Geometry: final body of the model. Coordinates: model frame, mm. Coordinates: 2 decimals unless noted, no trailing zeros. Loops run counter-clockwise (first coordinate to the right, second up) from the corner with the lowest first, then second, coordinate; pieces in that order, holes last. Notation, with made-up numbers: (53.5, 75.25) -> (90.5, 75.25) arc R26 cw to (90.5, 113.25) -> close; hole circle Ø7 at (31.25, -6). An arc over 180 degrees is marked (long way). One line per item, written item: value. Start each with the question number.
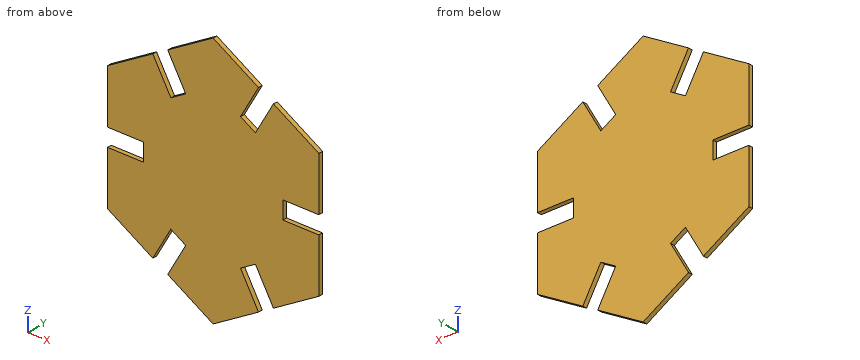
from build123d import *

# Parameters (mm, degrees)
BOSS_EXTRUDE1_DEPTH = 1.5875
SKETCH2_W           = 13.27114317
SKETCH2_H           = 6.35
CUT_EXTRUDE1_DEPTH  = 71.000903906


with BuildPart() as part:
    # Sketch1 → Boss-Extrude1 (new body)
    with BuildSketch(Plane(origin=(0, 0, 0), x_dir=(1, 0, 0), z_dir=(0, 1, 0))):
        Polygon((26.221215583, 24.643793134), (-12.749927587, 47.143793134), (-51.721070757, 24.643793134), (-51.721070757, -20.356206866), (-12.749927587, -42.856206866), (26.221215583, -20.356206866), align=None)
    extrude(amount=BOSS_EXTRUDE1_DEPTH)

    # Sketch2 → Cut-Extrude1 (cut, through all)
    with BuildSketch(Plane(origin=(0, 1.5875, 0), x_dir=(1, 0, 0), z_dir=(0, 1, 0))):
        with Locations((19.585643998, 2.143793134)):
            Rectangle(SKETCH2_W, SKETCH2_H)
        Polygon((2.84970307, 22.813146011), (9.485274655, 34.306293134), (3.986013341, 37.481293134), (-2.649558244, 25.988146011), align=None)
        Polygon((-22.85029693, 25.988146011), (-29.485868515, 37.481293134), (-34.985129829, 34.306293134), (-28.349558244, 22.813146011), align=None)
        with Locations((-45.085499172, 2.143793134)):
            Rectangle(SKETCH2_W, SKETCH2_H)
        Polygon((3.986013341, -33.193706866), (9.485274655, -30.018706866), (2.84970307, -18.525559743), (-2.649558244, -21.700559743), align=None)
        Polygon((-34.985129829, -30.018706866), (-29.485868515, -33.193706866), (-22.85029693, -21.700559743), (-28.349558244, -18.525559743), align=None)
    extrude(amount=-CUT_EXTRUDE1_DEPTH, mode=Mode.SUBTRACT)


solid = part.part
1. Line query: L1, parallel to X at y = 0.4, z = 29; L2, parallel to X at y = 1.15, z = 22; L3, parallel to Z at x = -2, y = 0.9. Output: solid intervals per line, ascending. Write a range as [from, to].
2. Pin query (flat end, axial travel): pin 1 Ø0.5 at (y, z) = (1, -2) entering from +X; pin 2 Ø0.8 at (x, y) = (20.5, 1) entering from +Z; pin 3 Ø0.5 at (x, y) = (19.5, 0.5) entering from -Z. Return the tip coordinate at first contact, or that it passes through.
3. Section D-D on x = -15.5. Return the cut outline in (y, z), plus the area to 3 significant figures.
4. Section C-C on z = -2.5. Return the cut outline in (x, y), plus the area to 3 significant figures.
5. Section B-B on x = 15. Return the cut outline in (y, z), plus the area to 3 significant figures.
Checks:
1. L1: [-36.75, -34.4], [-27.06, 1.56], [8.9, 11.25]
1. L2: [-48.87, -30.36], [-23.02, -2.48], [4.86, 23.37]
1. L3: [-40.94, -27.11], [-25.61, 21.33], [22.83, 36.65]
2. pin 1: x = 12.95
2. pin 2: z = 23.89
2. pin 3: z = -28.67
3. outline: (0, -45.56) -> (1.59, -45.56) -> (1.59, 41.27) -> (0, 41.27) -> close
3. area: 138 mm²
4. outline: (-38.45, 0) -> (12.95, 0) -> (12.95, 1.59) -> (-38.45, 1.59) -> close
4. area: 81.6 mm²
5. outline: (0, -31.12) -> (1.59, -31.12) -> (1.59, -5.32) -> (0, -5.32) -> close; (0, 1.03) -> (1.59, 1.03) -> (1.59, 26.83) -> (0, 26.83) -> close
5. area: 81.9 mm²
